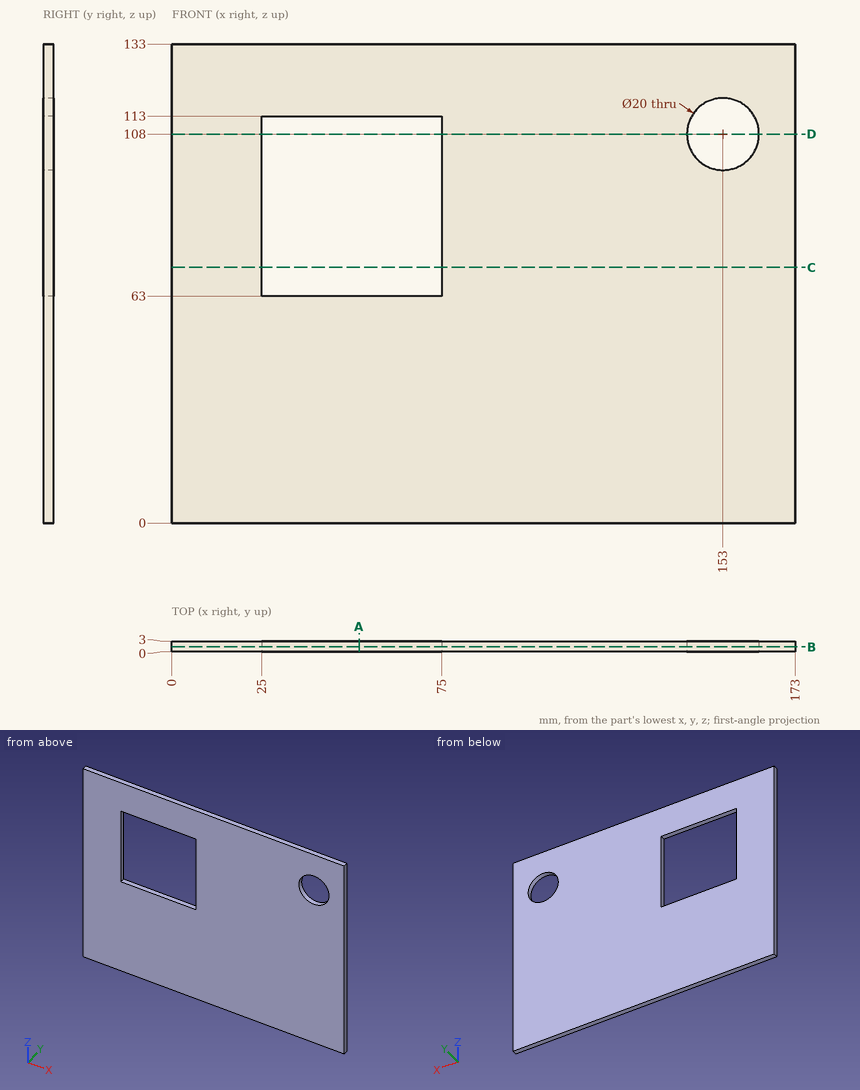
Verification items for this drawing (mm, ordinates from the low corner). Give positions to 0.01 mm unless a question says otherwise; leave off trailing zeros. Write each loop counter-clockwise with the first axis right and the second up, starting at its lowest first coordinate (ties: lowest second). Pieces come first, ordered by that corner, then holes. Notation, with made-up numbers: M 7,45.5 L 30,45.5 A21 cw 30,58.5 Z; hole C 33.5,-22 d1. An arc over 180 degrees is marked long. Use one line per item in the form item = value.
(1) Section check C-C on z = 71. Record the boundary of the cut face in (x, y).
Answer block:
outline = M 0,0 L 25,0 L 25,3 L 0,3 Z; M 75,0 L 173,0 L 173,3 L 75,3 Z
(2) Section check D-D on z = 108. Record the boundary of the cut face in (x, y), plus the area to 3 significant figures.
Answer block:
outline = M 0,0 L 25,0 L 25,3 L 0,3 Z; M 75,0 L 143,0 L 143,3 L 75,3 Z; M 163,0 L 173,0 L 173,3 L 163,3 Z
area = 309 mm2
(3) Section check A-A on x = 52. Record the boundary of the cut face in (y, z), plus the area to 3 significant figures.
Answer block:
outline = M 0,0 L 3,0 L 3,63 L 0,63 Z; M 0,113 L 3,113 L 3,133 L 0,133 Z
area = 249 mm2
(4) Section check B-B on y = 1.4. Record the boundary of the cut face in (x, z).
Answer block:
outline = M 0,0 L 173,0 L 173,133 L 0,133 Z; hole M 25,63 L 75,63 L 75,113 L 25,113 Z; hole C 153,108 d20
(5) Material ranges on line 1 along X through (y, z) = (1.4, 108); line 2 along X through (y, z) = (1.4, 91); line 3 along Z through (x, y) = (153, 1.4), recorded low to high.
Answer block:
line_1 = 0 to 25, 75 to 143, 163 to 173
line_2 = 0 to 25, 75 to 173
line_3 = 0 to 98, 118 to 133
